```python
from build123d import *

# Parameters (mm, degrees)
BOSS_EXTRUDE1_DEPTH = 2.5
SKETCH4_R           = 1.5
CUT_EXTRUDE1_DEPTH  = 5
SKETCH5_R           = 1.35
BOSS_EXTRUDE2_DEPTH = 0.6
SKETCH6_R           = 0.85
CUT_EXTRUDE3_DEPTH  = 1


with BuildPart() as part:
    # Sketch1 → Boss-Extrude1 (new, symmetric)
    with BuildSketch(Plane(origin=(0, 0, 0), x_dir=(1, 0, 0), z_dir=(0, 1, 0))):
        Polygon((4.041451884, 0), (2.020725942, 3.5), (-2.020725942, 3.5), (-4.041451884, 0), (-2.020725942, -3.5), (2.020725942, -3.5), align=None)
    extrude(amount=BOSS_EXTRUDE1_DEPTH, both=True)

    # Sketch2 → Cut-Revolve1 (revolve, cut)
    with BuildSketch(Plane.XY, mode=Mode.PRIVATE) as cut_revolve1_sk:
        Polygon((4.041451884, 2.5), (3.241451884, 2.5), (4.041451884, 1.9), align=None)
        Polygon((4.041451884, -2.5), (4.041451884, -1.9), (3.241451884, -2.5), align=None)
    revolve(cut_revolve1_sk.sketch.rotate(Axis((0, 2.5, 0), (0, -1, 0)), 90), axis=Axis((0, 2.5, 0), (0, -1, 0)), mode=Mode.SUBTRACT)

    # Sketch4 → Cut-Extrude1 (cut)
    with BuildSketch(Plane(origin=(0, 2.5, 0), x_dir=(1, 0, 0), z_dir=(0, 1, 0))):
        with Locations(Location((0, 0, 0), (0, 0, 270))):
            Circle(SKETCH4_R)
    extrude(amount=-CUT_EXTRUDE1_DEPTH, mode=Mode.SUBTRACT)

    # Sketch5 → Boss-Extrude2 (add)
    with BuildSketch(Plane(origin=(-3.031088913, 0, -1.75), x_dir=(-0.4999999999999951, 0, 0.8660254037844415), z_dir=(-0.8660254037844416, 0, -0.49999999999999517))):
        with Locations(Location((0, 0, 0), (0, 0, 180))):
            Circle(SKETCH5_R)
    extrude(amount=BOSS_EXTRUDE2_DEPTH)

    # Sketch6 → Cut-Extrude3 (cut)
    with BuildSketch(Plane(origin=(-3.550704156, 0, -2.05), x_dir=(-0.4999999999999952, 0, 0.8660254037844414), z_dir=(-0.8660254037844414, 0, -0.4999999999999952))):
        Circle(SKETCH6_R)
    extrude(amount=-CUT_EXTRUDE3_DEPTH, mode=Mode.SUBTRACT)


solid = part.part
```
CAD build for the part. Positions are in the model's coordinates, mm. A direction names the side the tool comes from. Coordinates: 2 decimals unless noted, no trailing zeros. Write each loop counter-clockwise with the first axis right and the second up, starting at its lowest first coordinate (ties: lowest second). Pieces come first, ordered by that corner, then holes.
(1) 3-axis set-ups, long thin cutter, end or side, ignore diameter. For faces 4 (the face through (-2.68, 0.01, -1.56)), 5 (the face through (0.7, -2.5, -1.5)): which of +Z, -Z, +X, -X, +Y, -Y reach the whole face in a straight line?
(2) Cut at C-C, the plane y = -1.05. List the corners of the cut face in (x, z), and give its area (3 significant figures).
(3) Flat gauge pins, fed straight in: pin 1 (2.5 mm diameter, centred on x = 0, z = 0, fed in from -Y); pin 2 (3 mm diameter, centred on y = 1.5, z = -2.5, fed in from +X); pin 3 (3 mm diameter, centred on x = -3, y = 1.5, fed in from -Z). Where does each tip first touch, or does it go through?
(4) Drill centre lines: probe 1 along X at (y, z) = (-0.4, -1); probe 2 along X at (y, z) = (1.95, -0.75); probe 3 along Z at (x, y) = (-0.5, 1.05). Where is each one in solid material? Low to high.
(5) Cut at B-B, the plane y = 1.8. List the corners of the cut face in (x, z).
(6) Two-plate mould, pull along Z, no slides. Class faces 1 (the face through (3.045, 0.032, -1.726)), 2 (the face through (-3.82, 0.82, -0.97)), 3 (the face through (-3.045, 0.032, 1.726)): +Z half, -Z half, draft (parallel to the pull), parting line (faces both ways), or undercut.
(7) Cut at A-A, the plane x = 0. List the corners of the cut face in (y, z), and give its area (3 significant figures).
(8) Cut at D-D, the plane y = -0.45. List the corners of the cut face in (x, z), and give its area (3 significant figures).
Geometry says:
1. face 4: none
1. face 5: +Z, -Z, +X, -X, -Y
2. outline: (-4.04, 0) - (-3.46, -1.02) - (-3.97, -1.32) - (-3.13, -2.78) - (-2.61, -2.48) - (-2.02, -3.5) - (2.02, -3.5) - (4.04, 0) - (2.02, 3.5) - (-2.02, 3.5) - close; hole circle Ø3 at (0, 0)
2. area: 36.4 mm2
3. pin 1: passes through
3. pin 2: stops at x = 3.46
3. pin 3: stops at z = -3.5
4. probe 1: x = -4.16 to -3.23, -3 to -1.12, 1.12 to 3.46
4. probe 2: x = -3.61 to -1.3, 1.3 to 3.61
4. probe 3: z = -3.5 to -1.41, 1.41 to 3.5
5. outline: (-4.04, 0) - (-2.02, -3.5) - (2.02, -3.5) - (4.04, 0) - (2.02, 3.5) - (-2.02, 3.5) - close; hole circle Ø3 at (0, 0)
6. face 1: -Z half
6. face 2: undercut
6. face 3: +Z half
7. outline: (-2.5, -3.24) - (-2.31, -3.5) - (2.31, -3.5) - (2.5, -3.24) - (2.5, -1.5) - (-2.5, -1.5) - close; (-2.5, 1.5) - (2.5, 1.5) - (2.5, 3.24) - (2.31, 3.5) - (-2.31, 3.5) - (-2.5, 3.24) - close
7. area: 19.9 mm2
8. outline: (-4.19, -0.95) - (-3.91, -1.43) - (-3.05, -0.93) - (-2.32, -2.17) - (-3.19, -2.67) - (-2.91, -3.15) - (-2.39, -2.85) - (-2.02, -3.5) - (2.02, -3.5) - (4.04, 0) - (2.02, 3.5) - (-2.02, 3.5) - (-4.04, 0) - (-3.67, -0.65) - close; hole circle Ø3 at (0, 0)
8. area: 35.5 mm2
